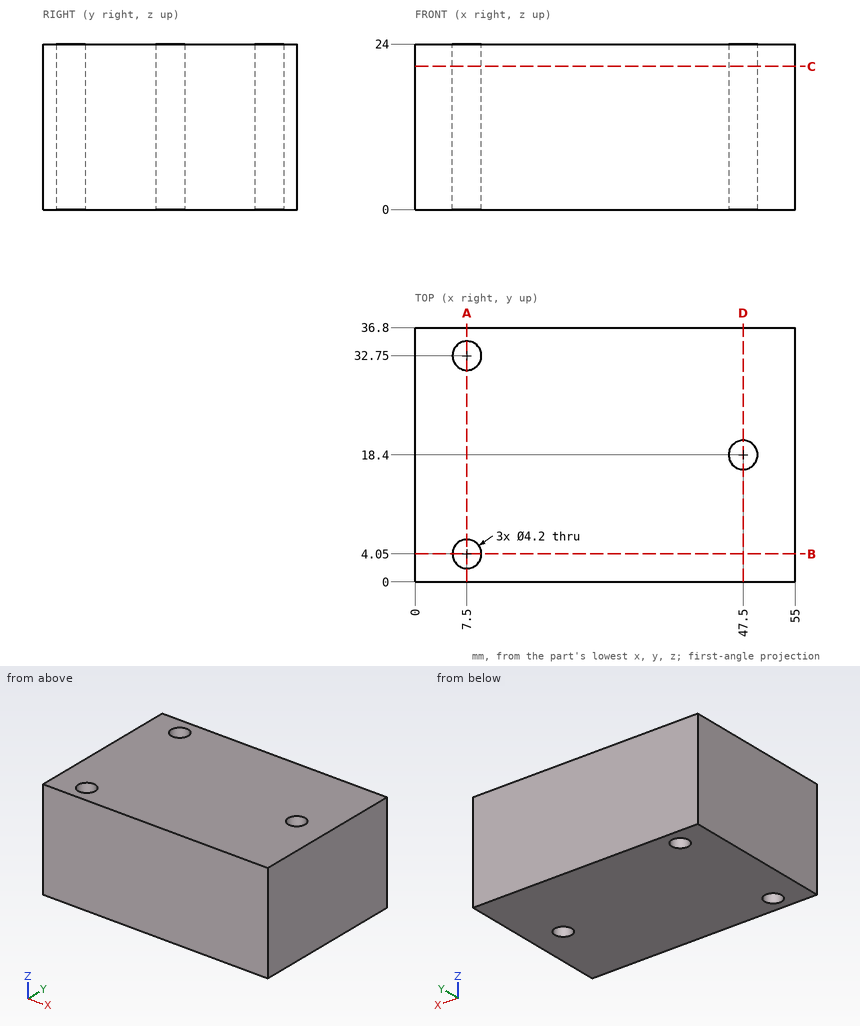
Geometry: see drawing. Coordinates: mm, zero at the bounding-box minimum. Give positions to 0.01 mm unless a question says otherwise; leave off trailing zeros. Loops run counter-clockwise (first coordinate to the right, second up) from the corner with the lowest first, then second, coordinate; pieces in that order, holes last. Notation, with made-up numbers: (-17.75, 28.25) - (-7.75, 28.25) arc R19 ccw to (-7.75, 61.25) - close; hole circle Ø2 at (82, -10.75). An arc over 180 degrees is marked (long way). Use CSV: the item, a comma, the result in double quotes. Start each with the question number.
1. Section C-C (z = 20.75). Output: boundary loops of the cut face in (x, y).
2. Section B-B (y = 4.05). Output: boundary loops of the cut face in (x, z).
3. Section A-A (x = 7.5). Output: boundary loops of the cut face in (y, z), then the cut area to 3 significant figures.
4. Section D-D (x = 47.5). Output: boundary loops of the cut face in (y, z).
5. Ray query, L1, parallel to Y at x = 7.5, z = 18.75; L2, parallel to Y at x = 47.5, z = 5.25; L3, parallel to X at y = 4.05, z = 8.5. Return the intervals inside material, ascending.
Response:
1,outline,"(0, 0) - (55, 0) - (55, 36.8) - (0, 36.8) - close; hole circle Ø4.2 at (7.5, 4.05); hole circle Ø4.2 at (7.5, 32.75); hole circle Ø4.2 at (47.5, 18.4)"
2,outline,"(0, 0) - (5.4, 0) - (5.4, 24) - (0, 24) - close; (9.6, 0) - (55, 0) - (55, 24) - (9.6, 24) - close"
3,outline,"(0, 0) - (1.95, 0) - (1.95, 24) - (0, 24) - close; (6.15, 0) - (30.65, 0) - (30.65, 24) - (6.15, 24) - close; (34.85, 0) - (36.8, 0) - (36.8, 24) - (34.85, 24) - close"
3,area,"682 mm²"
4,outline,"(0, 0) - (16.3, 0) - (16.3, 24) - (0, 24) - close; (20.5, 0) - (36.8, 0) - (36.8, 24) - (20.5, 24) - close"
5,L1,"0 to 1.95, 6.15 to 30.65, 34.85 to 36.8"
5,L2,"0 to 16.3, 20.5 to 36.8"
5,L3,"0 to 5.4, 9.6 to 55"
